Verification items for the finished model (mm, model axes). A direction names the side the tool comes from. Give positions to 0.01 mm unless a question says otherwise; leave off trailing zeros. Write each loop counter-clockwise with the first axis right and the second up, starting at its lowest first coordinate (ties: lowest second). Pieces come first, ordered by that corner, then holes. Notation, with made-up numbers: (60.5, 85.5) -> (84.5, 85.5) arc R17 cw to (84.5, 92.5) -> close; hole circle Ø1 at (6.25, -25). An arc over 180 degrees is marked (long way). Answer as CSV lines item,"result". Start each with the question number.
1) Sectioned sample at B-B on z = 9. Record the cut outline in (x, y), and give its area (3 significant figures).
2) Sectioned sample at A-A on y = 25. Record the cut outline in (x, z).
3) Sectioned sample at C-C on x = -13. Record the cut outline in (y, z), and give its area (3 significant figures).
4) Material ranges on L1, parallel to X at y = 12, z = 4.5; L2, parallel to X at y = 24, z = 1.25; L3, parallel to Z at x = 15, y = 31, recorded low to high.
5) Mould release check, pull along X, two halves, no side actions. Record for faces 4 (the flat face through (-22, 3, 16)), 5 (the cylindrical face through (10.6, 23.2, 3)), 6 (the flat face through (-21.7, 5.814, 10.93)), 7 (the cylindrical face through (-24.78, 3.31, 10.93)): released by +X, released by -X, zero draft, split by the parting line, or undercut.
6) Gauge pin test, flat ends, axial feed: pin 1 Ø15 at (x, y) = (10.5, 37.5) entering from +Z; pin 2 Ø8 at (x, z) = (-14.5, 13.5) entering from +Y; pin 3 Ø4 at (x, z) = (1.5, 7) entering from -Y. Record the tip position at first contact, or that the pin passes through.
7) Tool access check on faces 1 (the flat face through (21.767, 5.832, 10.93)), 2 (the cylindrical face through (24.79, 3.22, 10.93)), 3 (the flat face through (-25, 25, 3)). Record the directions out of +Z, -Z, +X, -X, +Y, -Y that give a thin tool (end or side, any length) a straight path to the whole face; none if there is none.
8) Sectioned sample at D-D on z = 4.5. Record the cut outline in (x, y).
```python
from build123d import *

# Parameters (mm, degrees)
BOSS_EXTRUDE1_DEPTH = 6
BOSS_EXTRUDE2_DEPTH = 10
BOSS_EXTRUDE3_DEPTH = 6
SKETCH4_R           = 3
CUT_EXTRUDE1_DEPTH  = 57.789083458


with BuildPart() as part:
    # Sketch1 → Boss-Extrude1 (new body)
    with BuildSketch(Plane.XY):
        with BuildLine():
            Line((20, 0), (25, 0))
            ThreePointArc((25, 0), (0, 25), (-25, 0))
            Line((-25, 0), (-20, 0))
            ThreePointArc((-20, 0), (0, 20), (20, 0))
        make_face()
    extrude(amount=BOSS_EXTRUDE1_DEPTH)

    # Sketch2 → Boss-Extrude2 (add)
    with BuildSketch(Plane.XY.offset(6)):
        with BuildLine():
            ThreePointArc((-20, 0), (-19.828897227, 2.610523844), (-19.318516526, 5.176380902))
            Line((-19.318516526, 5.176380902), (-24.148145657, 6.470476128))
            ThreePointArc((-24.148145657, 6.470476128), (-24.786121534, 3.263154806), (-25, 0))
            Line((-25, 0), (-20, 0))
        make_face()
        with BuildLine():
            Line((24.148145657, 6.470476128), (19.318516526, 5.176380902))
            ThreePointArc((19.318516526, 5.176380902), (19.828897227, 2.610523844), (20, 0))
            Line((20, 0), (25, 0))
            ThreePointArc((25, 0), (24.786121534, 3.263154806), (24.148145657, 6.470476128))
        make_face()
    extrude(amount=BOSS_EXTRUDE2_DEPTH)

    # Sketch3 → Boss-Extrude3 (add)
    with BuildSketch(Plane(origin=(0, 0, 0), x_dir=(-1, 0, 0), z_dir=(0, 0, -1))):
        with BuildLine():
            Line((-25, 0), (-25, 50))
            Line((-25, 50), (25, 50))
            Line((25, 50), (25, 0))
            ThreePointArc((25, 0), (0, 25), (-25, 0))
        make_face()
    extrude(amount=-BOSS_EXTRUDE3_DEPTH)

    # Sketch4 → Cut-Extrude1 (cut, through all)
    with BuildSketch(Plane.XY.offset(6)):
        with Locations((13, 25)):
            Circle(SKETCH4_R)
        with Locations((-13, 25)):
            Circle(SKETCH4_R)
    extrude(amount=-CUT_EXTRUDE1_DEPTH, mode=Mode.SUBTRACT)


solid = part.part
```
Ans:
1,outline,"(-25, 0) -> (-20, 0) arc R20 cw to (-19.32, 5.18) -> (-24.15, 6.47) arc R25 ccw to start; (19.32, 5.18) arc R20 cw to (20, 0) -> (25, 0) arc R25 ccw to (24.15, 6.47) -> close"
1,area,"58.9 mm²"
2,outline,"(-25, 0) -> (-16, 0) -> (-16, 6) -> (-25, 6) -> close; (-10, 0) -> (10, 0) -> (10, 6) -> (-10, 6) -> close; (16, 0) -> (25, 0) -> (25, 6) -> (16, 6) -> close"
3,outline,"(15.2, 0) -> (22, 0) -> (22, 6) -> (15.2, 6) -> close; (28, 0) -> (50, 0) -> (50, 6) -> (28, 6) -> close"
3,area,"173 mm²"
4,L1,"x = -25 to -16, 16 to 25"
4,L2,"x = -25 to -15.83, -10.17 to 10.17, 15.83 to 25"
4,L3,"z = 0 to 6"
5,face 4,"zero draft"
5,face 5,"undercut"
5,face 6,"undercut"
5,face 7,"released by -X"
6,pin 1,"stops at z = 6"
6,pin 2,"passes through"
6,pin 3,"stops at y = 19.74"
7,face 1,"+Z, +Y"
7,face 2,"+Z, +X, +Y"
7,face 3,"+Z, -Z, -X, +Y, -Y"
8,outline,"(-25, 0) -> (-20, 0) arc R20 cw to (20, 0) -> (25, 0) -> (25, 50) -> (-25, 50) -> close; hole circle Ø6 at (-13, 25); hole circle Ø6 at (13, 25)"
